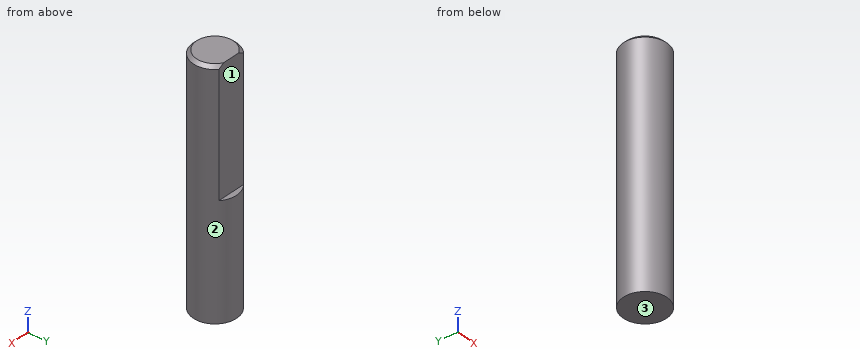
from build123d import *

# Parameters (mm, degrees)
ESQUISSE1_R             = 2
BOSS_EXTRU_1_DEPTH      = 12
BOSS_EXTRU_1_DEPTH_BACK = 10
CHANFREIN1_SIZE         = 0.3
ESQUISSE2_W             = 2.645751312
ESQUISSE2_H             = 0.5
ENL_V_MAT_EXTRU_1_DEPTH = 11.5


with BuildPart() as part:
    # Esquisse1 → Boss.-Extru.1 (new body, two sides)
    with BuildSketch(Plane.XY) as boss_extru_1_sk:
        Circle(ESQUISSE1_R)
    extrude(amount=BOSS_EXTRU_1_DEPTH)
    extrude(boss_extru_1_sk.sketch, amount=-BOSS_EXTRU_1_DEPTH_BACK)

    # Chanfrein1
    chanfrein1_edges = [part.edges().sort_by_distance(p)[0] for p in [
        (-2, 0, 12),
    ]]
    chamfer(chanfrein1_edges, length=CHANFREIN1_SIZE)

    # Esquisse2 → Enlèv. mat.-Extru.1 (cut)
    with BuildSketch(Plane.XY.offset(12)):
        with Locations((0, 1.75)):
            Rectangle(ESQUISSE2_W, ESQUISSE2_H)
    extrude(amount=-ENL_V_MAT_EXTRU_1_DEPTH, mode=Mode.SUBTRACT)


solid = part.part
Could you check a few things on this model? Use its own coordinates, in mm. Face numbers are marked on the shaded views. Coordinates: 2 decimals unless noted, no trailing zeros. Loops run counter-clockwise (first coordinate to the right, second up) from the corner with the lowest first, then second, coordinate; pieces in that order, holes last. Notation, with made-up numbers: (-14.75, -12.5) -> (6.25, -12.5) arc R14 cw to (6.25, 3.5) -> close; hole circle Ø3 at (32.25, 77.5). An arc over 180 degrees is marked (long way). Answer in a Markdown table with one row per item.
(1) Imagine slicing it at D-D (z = -5.25). List the corners of the cut face in (x, y) for me.
Results found:
| item | result |
|---|---|
| outline | circle Ø4 at (0, 0) |
(2) Thinking about a two-plate mould opening in Y: for the marked faces 1, 2 and 3, which applies, released by +Y, released by -Y, zero draft, split by the parting line, or undercut?
Results found:
| item | result |
|---|---|
| face 1 | released by +Y |
| face 2 | split by the parting line |
| face 3 | zero draft |
(3) Imagine slicing it at B-B (z = 8.75). List the corners of the cut face in (x, y) for me.
Results found:
| item | result |
|---|---|
| outline | (-1.32, 1.5) arc R2 ccw (long way) to (1.32, 1.5) -> close |
(4) Imagine slicing it at A-A (x = 0). List the corners of the cut face in (y, z) for me.
Results found:
| item | result |
|---|---|
| outline | (-2, -10) -> (2, -10) -> (2, 0.5) -> (1.5, 0.5) -> (1.5, 12) -> (-1.7, 12) -> (-2, 11.7) -> close |
(5) If I drill on probe 1 along Y at (x, z) = (1.5, 10); probe 2 along Z at (x, y) = (0.55, 1.6); probe 3 along Y at (x, z) = (0.05, 4), over which ranges is the centre line in solid material (lowest first)?
Results found:
| item | result |
|---|---|
| probe 1 | y = -1.32 to 1.32 |
| probe 2 | z = -10 to 0.5 |
| probe 3 | y = -2 to 1.5 |
(6) Imagine slicing it at C-C (y = 1.75). List the corners of the cut face in (x, z) for me, plus the area to 3 significant figures.
Results found:
| item | result |
|---|---|
| outline | (-0.97, -10) -> (0.97, -10) -> (0.97, 0.5) -> (-0.97, 0.5) -> close |
| area | 20.3 mm^2 |
